CAD build for the part. Positions are in the model's coordinates, mm. A direction names the side the tool comes from. Give positions to 0.01 mm unless a question says otherwise; leave off trailing zeros. Loops run counter-clockwise (first coordinate to the right, second up) from the corner with the lowest first, then second, coordinate; pieces in that order, holes last. Notation, with made-up numbers: M 67.5,58.5 L 95.5,58.5 A17 ccw 95.5,84.5 Z; hole C 83,59 d1. An arc over 180 degrees is marked long. One line per question, with ' | ' between items.
```python
from build123d import *

# Parameters (mm, degrees)
BOSS_EXTRUDE1_DEPTH        = 12.065
FILLET2_R                  = 1.27
FILLET3_R                  = 1.27
CUT_EXTRUDE1_REACH         = 41.898
F_5_0_5_DIAMETER_HOLE1_D   = 5
CUT_EXTRUDE2_DEPTH         = 2.159
CUT_EXTRUDE3_DEPTH         = 4.699
F_97_0_22_DIAMETER_HOLE1_D = 5.588
SKETCH12_R                 = 6.477
CUT_EXTRUDE4_DEPTH         = 1.778
M2X0_4_TAPPED_HOLE1_D      = 2
M2X0_4_TAPPED_HOLE1_DEPTH  = 4.2418
M2X0_4_TAPPED_HOLE1_TIP    = 0.600860619


with BuildPart() as part:
    # Sketch1 → Boss-Extrude1 (new body)
    with BuildSketch(Plane(origin=(0, 0, 0), x_dir=(1, 0, 0), z_dir=(0, 1, 0))):
        with BuildLine():
            Line((20.955, 9.017), (20.955, 4.826))
            Line((20.955, 4.826), (34.29, 4.826))
            Line((34.29, 4.826), (34.29, -4.826))
            Line((34.29, -4.826), (20.955, -4.826))
            Line((20.955, -4.826), (20.955, -9.017))
            Line((20.955, -9.017), (1.484742221, -11.525257515))
            ThreePointArc((1.484742221, -11.525257515), (-11.6205, 0), (1.484742221, 11.525257515))
            Line((1.484742221, 11.525257515), (20.955, 9.017))
        make_face()
    extrude(amount=BOSS_EXTRUDE1_DEPTH)

    # Fillet2
    fillet2_edges = [part.edges().sort_by_distance(p)[0] for p in [
        (20.955, 6.0325, 4.826),
    ]]
    fillet(fillet2_edges, radius=FILLET2_R)

    # Fillet3
    fillet3_edges = [part.edges().sort_by_distance(p)[0] for p in [
        (20.955, 6.0325, -4.826),
    ]]
    fillet(fillet3_edges, radius=FILLET3_R)

    # Sketch3 → Cut-Extrude1 (cut, up to next)
    with BuildSketch(Plane(origin=(0, 0, -4.826), x_dir=(-1, 0, 0), z_dir=(0, 0, -1)), mode=Mode.PRIVATE) as cut_extrude1_sk1:
        with BuildLine():
            ThreePointArc((-34.29, 6.0325), (-32.523121658, 10.298121658), (-28.2575, 12.065))
            Line((-28.2575, 12.065), (-34.29, 12.065))
            Line((-34.29, 12.065), (-34.29, 6.0325))
        make_face()
    cut_extrude1_tool1 = extrude(cut_extrude1_sk1.sketch, amount=-CUT_EXTRUDE1_REACH, mode=Mode.PRIVATE) & part.part
    # Sketch3 → Cut-Extrude1 (cut, up to next)
    with BuildSketch(Plane(origin=(0, 0, -4.826), x_dir=(-1, 0, 0), z_dir=(0, 0, -1)), mode=Mode.PRIVATE) as cut_extrude1_sk2:
        with BuildLine():
            ThreePointArc((-28.2575, 0), (-32.523121658, 1.766878342), (-34.29, 6.0325))
            Line((-34.29, 6.0325), (-34.29, 0))
            Line((-34.29, 0), (-28.2575, 0))
        make_face()
    cut_extrude1_tool2 = extrude(cut_extrude1_sk2.sketch, amount=-CUT_EXTRUDE1_REACH, mode=Mode.PRIVATE) & part.part
    add(cut_extrude1_tool1.solids().sort_by_distance((32.942533, 10.717533, -4.826))[0], mode=Mode.SUBTRACT)
    add(cut_extrude1_tool2.solids().sort_by_distance((32.942533, 1.347467, -4.826))[0], mode=Mode.SUBTRACT)

    # Ø5.0 (5) Diameter Hole1 (through all)
    with Locations(Plane.XY.offset(4.826)):
        with Locations((29.972, 6.0325)):
            Hole(F_5_0_5_DIAMETER_HOLE1_D / 2)

    # Sketch8 → Cut-Extrude2 (cut)
    with BuildSketch(Plane(origin=(0, 12.065, 0), x_dir=(1, 0, 0), z_dir=(0, 1, 0))):
        with BuildLine():
            ThreePointArc((4.828317518, 8.284122295), (-9.5885, 0), (4.828317518, -8.284122295))
            ThreePointArc((4.828317518, -8.284122295), (17.8435, 0), (4.828317518, 8.284122295))
        make_face()
    extrude(amount=-CUT_EXTRUDE2_DEPTH, mode=Mode.SUBTRACT)

    # Sketch9 → Cut-Extrude3 (cut)
    with BuildSketch(Plane(origin=(0, 9.906, 0), x_dir=(1, 0, 0), z_dir=(0, 1, 0))):
        with BuildLine():
            ThreePointArc((6.995671394, 5.588), (-8.9535, 0), (6.995671394, -5.588))
            ThreePointArc((6.995671394, -5.588), (11.975498152, -4.059363478), (15.24, 0))
            ThreePointArc((15.24, 0), (11.975498152, 4.059363478), (6.995671394, 5.588))
        make_face()
    extrude(amount=-CUT_EXTRUDE3_DEPTH, mode=Mode.SUBTRACT)

    # #97 (0.22) Diameter Hole1 (through all)
    with Locations(Plane(origin=(0, 0, 0), x_dir=(-1, 0, 0), z_dir=(0, -1, 0))):
        with Locations((-14.605, 0)):
            Hole(F_97_0_22_DIAMETER_HOLE1_D / 2)

    # Sketch12 → Cut-Extrude4 (cut)
    with BuildSketch(Plane(origin=(0, 5.207, 0), x_dir=(1, 0, 0), z_dir=(0, 1, 0))):
        with Locations(Location((0, 0, 0), (0, 0, 270))):
            Circle(SKETCH12_R)
    extrude(amount=-CUT_EXTRUDE4_DEPTH, mode=Mode.SUBTRACT)

    # M2x0.4 Tapped Hole1
    with Locations(Plane(origin=(0, 9.906, 0), x_dir=(1, 0, 0), z_dir=(0, 1, 0))):
        with Locations((8.6995, 6.985), (8.6995, -6.985)):
            Hole(M2X0_4_TAPPED_HOLE1_D / 2, depth=M2X0_4_TAPPED_HOLE1_DEPTH)
            with Locations((0, 0, -(M2X0_4_TAPPED_HOLE1_DEPTH + M2X0_4_TAPPED_HOLE1_TIP / 2))):  # 118° drill point
                Cone(0, M2X0_4_TAPPED_HOLE1_D / 2, M2X0_4_TAPPED_HOLE1_TIP, mode=Mode.SUBTRACT)


solid = part.part
```
Item 1: Saw through at C-C on x = 0. Give the cut face in (y, z) (1 decimal).
Conclusion:
outline: M 0,-11.6 L 12.1,-11.6 L 12.1,-9.6 L 9.9,-9.6 L 9.9,-9 L 5.2,-9 L 5.2,-6.5 L 3.4,-6.5 L 3.4,6.5 L 5.2,6.5 L 5.2,9 L 9.9,9 L 9.9,9.6 L 12.1,9.6 L 12.1,11.6 L 0,11.6 Z
Item 2: Drop flat-ended pins along their axis: P1, Ø3, axis at x = 8.7, z = 6.98, coming from the +Y side; P2, Ø1.5, axis at x = 1, y = 4, coming from the +Z side; P3, Ø8, axis at x = 0, z = 0, coming from the +Y side. Give the stop position or say it passes through.
Conclusion:
P1: y = 9.91 | P2: z = 11.62 | P3: y = 3.43
Item 3: Saw through at B-B on y = 7.5. Give the cut face in (x, z) (1 decimal), and give its area (3 significant figures).
Conclusion:
outline: M 1.5,-11.5 L 21,-9 L 21,-6.1 A1.3 cw 22.2,-4.8 L 27.9,-4.8 L 27.9,4.8 L 22.2,4.8 A1.3 cw 21,6.1 L 21,9 L 1.5,11.5 A11.6 ccw long Z; M 32,-4.8 L 34.1,-4.8 L 34.1,4.8 L 32,4.8 Z; hole M 7,-5.6 A8.9 ccw 13.6,-2.6 A2.8 ccw long 13.6,2.6 A8.9 ccw 7,5.6 A9 ccw long Z; hole C 8.7,-7 d2; hole C 8.7,7 d2 | area: 412 mm²
Item 4: Mould opens along X. For faces 1 (the cylindrical face through (10.58, 7.59, 4.83)), 2 (the flat face through (11.356, 5.948, 10.254)) say: pulls with the +X half, pulls with the -X half, needs draft (parallel to the pull), parting line crosses it, or undercut.
Conclusion:
face 1: undercut | face 2: pulls with the +X half
Item 5: Saw through at A-A on z = 0. Give the cut face in (x, y) (1 decimal), and give its area (3 significant figures).
Conclusion:
outline: M -11.6,0 L 11.8,0 L 11.8,5.2 L 6.5,5.2 L 6.5,3.4 L -6.5,3.4 L -6.5,5.2 L -9,5.2 L -9,9.9 L -9.6,9.9 L -9.6,12.1 L -11.6,12.1 Z; M 17.4,0 L 28.3,0 A6 ccw 28.3,12.1 L 17.8,12.1 L 17.8,9.9 L 17.4,9.9 Z; hole C 30,6 d5 | area: 283 mm²
Item 6: Drill centre lines: line 1 along X through (y, z) = (6.25, -1.75); line 2 along Y through (x, z) = (13, -7.25); line 3 along X through (y, z) = (4.25, -3.25). Where is each one in solid material? Low to high. Write a range as [from, to].
Conclusion:
line 1: [-11.49, -8.78], [16.78, 27.48], [32.46, 34.29] | line 2: [0, 9.91] | line 3: [-11.16, -5.6], [5.6, 28.22], [31.72, 34.02]
Item 7: 3-axis set-ups, long thin cutter, end or side, ignore diameter. For faces 3 (the flat face through (20.955, 6, 8)), 4 (the cylindrical face through (8.162, 7.755, -7.828)), 5 (the flat face through (20.955, 6, -8)): which of +Z, -Z, +X, -X, +Y, -Y reach the whole face in a straight line?
Conclusion:
face 3: +Z, +X, +Y, -Y | face 4: +Y | face 5: -Z, +X, +Y, -Y
Item 8: Saw through at D-D on y = 11.25. Give the cut face in (x, z) (1 decimal).
Conclusion:
outline: M 1.5,-11.5 L 21,-9 L 21,-6.1 A1.3 cw 22.2,-4.8 L 31.3,-4.8 L 31.3,4.8 L 22.2,4.8 A1.3 cw 21,6.1 L 21,9 L 1.5,11.5 A11.6 ccw long Z; hole M 4.8,-8.3 A9.1 ccw long 4.8,8.3 A9.6 ccw long Z
